Verification items for the finished model (mm, model axes). Round coordinates to 2 decimals unless told otherwise and drop trailing zeros. Order: outer loops, then holes, each group sorted by start corner. A loop starts at its lowest first (then second) coordinate and runs counter-clockwise, first axis right, second up. Notation, with made-up numbers: (-13.5, 14.5) -> (18.5, 14.5) arc R19 cw to (18.5, 45.5) -> close; hole circle Ø9 at (59.25, 33.5). An arc over 180 degrees is marked (long way). Put each result on its own line as item: value.
from build123d import *

# Parameters (mm, degrees)
BOSS_EXTRUDE1_DEPTH       = 0.3175
F_0_CLEARANCE_HOLE1_D     = 1.6129
F_0_CLEARANCE_HOLE1_DEPTH = 6.35
F_0_CLEARANCE_HOLE1_TIP   = 0.676691898


with BuildPart() as part:
    # Sketch1 → Boss-Extrude1 (new body)
    with BuildSketch(Plane(origin=(0, 0, 0), x_dir=(1, 0, 0), z_dir=(0, 1, 0))):
        with BuildLine():
            ThreePointArc((1.736526379, 0), (1.905, 0.168473621), (2.073473621, 0))
            Line((2.073473621, 0), (3.81, 0))
            Line((3.81, 0), (3.81, 1.905))
            Line((3.81, 1.905), (-3.81, 1.905))
            Line((-3.81, 1.905), (-3.81, 0))
            Line((-3.81, 0), (-2.064971223, 0))
            ThreePointArc((-2.064971223, 0), (-1.905, 0.159971223), (-1.745028777, 0))
            Line((-1.745028777, 0), (-0.8, 0))
            Line((-0.8, 0), (-0.8, 0.254))
            Line((-0.8, 0.254), (0.8, 0.254))
            Line((0.8, 0.254), (0.8, 0))
            Line((0.8, 0), (1.736526379, 0))
        make_face()
        with BuildLine():
            Line((3.81, 0), (2.073473621, 0))
            ThreePointArc((2.073473621, 0), (1.905, -0.168473621), (1.736526379, 0))
            Line((1.736526379, 0), (0.8, 0))
            Line((0.8, 0), (0.8, -0.254))
            Line((0.8, -0.254), (-0.8, -0.254))
            Line((-0.8, -0.254), (-0.8, 0))
            Line((-0.8, 0), (-1.745028777, 0))
            ThreePointArc((-1.745028777, 0), (-1.905, -0.159971223), (-2.064971223, 0))
            Line((-2.064971223, 0), (-3.81, 0))
            Line((-3.81, 0), (-3.81, -1.905))
            Line((-3.81, -1.905), (3.81, -1.905))
            Line((3.81, -1.905), (3.81, 0))
        make_face()
    extrude(amount=BOSS_EXTRUDE1_DEPTH)

    # #0 Clearance Hole1
    with Locations(Plane(origin=(-1.905, 0.3175, 0), x_dir=(0, 0, 1), z_dir=(0, 1, 0))):
        with Locations((0, 0), (0, 3.81)):
            Hole(F_0_CLEARANCE_HOLE1_D / 2, depth=F_0_CLEARANCE_HOLE1_DEPTH)
            with Locations((0, 0, -(F_0_CLEARANCE_HOLE1_DEPTH + F_0_CLEARANCE_HOLE1_TIP / 2))):  # 100° drill point
                Cone(0, F_0_CLEARANCE_HOLE1_D / 2, F_0_CLEARANCE_HOLE1_TIP, mode=Mode.SUBTRACT)


solid = part.part
Item 1: Section check C-C on y = 0.25. Record the boundary of the cut face in (x, z) (3 decimals).
Check sheet entries:
outline: (-3.81, -1.905) -> (3.81, -1.905) -> (3.81, 1.905) -> (-3.81, 1.905) -> close; hole circle Ø1.613 at (-1.905, 0); hole (-0.8, -0.254) -> (0.8, -0.254) -> (0.8, 0.254) -> (-0.8, 0.254) -> close; hole circle Ø1.613 at (1.905, 0)
Item 2: Gauge pin test, flat end, axial feed: pin 1 Ø2 at (x, z) = (-2.5, 0) entering from -Y. Record the tip position at first contact, or that the pin passes through.
Check sheet entries:
pin 1: stops at y = 0
Item 3: Material ranges on L1, parallel to X at y = 0.2, z = 0; L2, parallel to X at y = 0.1, z = 0.55; L3, parallel to Z at x = 2, y = 0.25 (3 decimals), recorded low to high. Write a range as [from, to].
Check sheet entries:
L1: x = [-3.81, -2.71], [-1.1, -0.8], [0.8, 1.1], [2.71, 3.81]
L2: x = [-3.81, -2.49], [-1.32, 1.32], [2.49, 3.81]
L3: z = [-1.905, -0.801], [0.801, 1.905]
Item 4: Section check D-D on z = 0.6. Record the boundary of the cut face in (x, y), then the cut area to 3 significant figures.
Check sheet entries:
outline: (-3.81, 0) -> (-2.44, 0) -> (-2.44, 0.32) -> (-3.81, 0.32) -> close; (-1.37, 0) -> (1.37, 0) -> (1.37, 0.32) -> (-1.37, 0.32) -> close; (2.44, 0) -> (3.81, 0) -> (3.81, 0.32) -> (2.44, 0.32) -> close
area: 1.74 mm^2
Item 5: Section check A-A on z = 0. Record the boundary of the cut face in (x, y).
Check sheet entries:
outline: (-3.81, 0) -> (-2.71, 0) -> (-2.71, 0.32) -> (-3.81, 0.32) -> close; (-1.1, 0) -> (-0.8, 0) -> (-0.8, 0.32) -> (-1.1, 0.32) -> close; (0.8, 0) -> (1.1, 0) -> (1.1, 0.32) -> (0.8, 0.32) -> close; (2.71, 0) -> (3.81, 0) -> (3.81, 0.32) -> (2.71, 0.32) -> close
Item 6: Release check for a two-part mould opening along X. For faces 1 (the cylindrical face through (-1.105, 0.157, 0.105)), 2 (the flat face through (-0.1, 0.318, -0.5)), 3 (the cylindrical face through (1.118, 0.157, 0.175)) record: +X half, -X half, draft (parallel to the pull), parting line (faces both ways), or undercut.
Check sheet entries:
face 1: undercut
face 2: draft
face 3: undercut
